```python
from build123d import *

# Parameters (mm, degrees)
F1_DEPTH = 1.5
F2_R     = 6
F3_R     = 20


with BuildPart() as f1:
    # F0 (on Top) → F1 (new body)
    with BuildSketch(Plane.XY):
        Polygon((16.235917, 84.775943), (-13.764083, 84.775943), (-13.764083, 61.775943), (-7.764083, 24.775943), (-7.764083, 9.775943), (-13.764083, -27.224057), (-13.764083, -50.224057), (16.235917, -50.224057), (16.235917, -27.224057), (10.235917, 9.775943), (10.235917, 24.775943), (16.235917, 61.775943), align=None)
        with BuildLine():
            ThreePointArc((-4.764083, -43.224057), (-4.471189, -42.51695), (-3.764083, -42.224057))
            Line((-3.764083, -42.224057), (6.235917, -42.224057))
            ThreePointArc((6.235917, -42.224057), (6.943024, -42.51695), (7.235917, -43.224057))
            ThreePointArc((7.235917, -43.224057), (6.943024, -43.931164), (6.235917, -44.224057))
            Line((6.235917, -44.224057), (-3.764083, -44.224057))
            ThreePointArc((-3.764083, -44.224057), (-4.471189, -43.931164), (-4.764083, -43.224057))
        make_face(mode=Mode.SUBTRACT)
        with BuildLine():
            Line((6.735917, 28.275943), (-3.764083, 28.275943))
            ThreePointArc((-3.764083, 28.275943), (-4.471189, 27.98305), (-4.764083, 27.275943))
            Line((-4.764083, 27.275943), (-4.764083, 19.275943))
            ThreePointArc((-4.764083, 19.275943), (-4.471189, 18.568836), (-3.764083, 18.275943))
            Line((-3.764083, 18.275943), (6.735917, 18.275943))
            ThreePointArc((6.735917, 18.275943), (7.089471, 18.129496), (7.235917, 17.775943))
            Line((7.235917, 17.775943), (7.235917, 17.275943))
            Line((7.235917, 17.275943), (7.235917, 16.775943))
            ThreePointArc((7.235917, 16.775943), (7.089471, 16.42239), (6.735917, 16.275943))
            Line((6.735917, 16.275943), (-3.764083, 16.275943))
            ThreePointArc((-3.764083, 16.275943), (-4.471189, 15.98305), (-4.764083, 15.275943))
            Line((-4.764083, 15.275943), (-4.764083, 7.275943))
            ThreePointArc((-4.764083, 7.275943), (-4.471189, 6.568836), (-3.764083, 6.275943))
            Line((-3.764083, 6.275943), (6.735917, 6.275943))
            ThreePointArc((6.735917, 6.275943), (7.089471, 6.129496), (7.235917, 5.775943))
            ThreePointArc((7.235917, 5.775943), (7.089471, 5.42239), (6.735917, 5.275943))
            Line((6.735917, 5.275943), (-4.764083, 5.275943))
            ThreePointArc((-4.764083, 5.275943), (-5.471189, 5.568836), (-5.764083, 6.275943))
            Line((-5.764083, 6.275943), (-5.764083, 16.775943))
            Line((-5.764083, 16.775943), (-5.764083, 17.775943))
            Line((-5.764083, 17.775943), (-5.764083, 28.275943))
            ThreePointArc((-5.764083, 28.275943), (-5.471189, 28.98305), (-4.764083, 29.275943))
            Line((-4.764083, 29.275943), (6.735917, 29.275943))
            ThreePointArc((6.735917, 29.275943), (7.089471, 29.129496), (7.235917, 28.775943))
            ThreePointArc((7.235917, 28.775943), (7.089471, 28.42239), (6.735917, 28.275943))
        make_face(mode=Mode.SUBTRACT)
        with BuildLine():
            Line((6.235917, 76.775943), (-3.764083, 76.775943))
            ThreePointArc((-3.764083, 76.775943), (-4.471189, 77.068836), (-4.764083, 77.775943))
            ThreePointArc((-4.764083, 77.775943), (-4.471189, 78.48305), (-3.764083, 78.775943))
            Line((-3.764083, 78.775943), (6.235917, 78.775943))
            ThreePointArc((6.235917, 78.775943), (6.943024, 78.48305), (7.235917, 77.775943))
            ThreePointArc((7.235917, 77.775943), (6.943024, 77.068836), (6.235917, 76.775943))
        make_face(mode=Mode.SUBTRACT)
    extrude(amount=F1_DEPTH)

    # F2
    f2_edges = [f1.edges().sort_by_distance(p)[0] for p in [
        (16.235917, 84.775943, 0.75),
        (-13.764083, 84.775943, 0.75),
        (-13.764083, -50.224057, 0.75),
        (16.235917, -50.224057, 0.75),
    ]]
    fillet(f2_edges, radius=F2_R)

    # F3
    f3_edges = [f1.edges().sort_by_distance(p)[0] for p in [
        (16.235917, 61.775943, 0.75),
        (-13.764083, 61.775943, 0.75),
        (16.235917, -27.224057, 0.75),
        (-13.764083, -27.224057, 0.75),
        (-7.764083, 9.775943, 0.75),
        (10.235917, 9.775943, 0.75),
        (10.235917, 24.775943, 0.75),
        (-7.764083, 24.775943, 0.75),
    ]]
    fillet(f3_edges, radius=F3_R)


solid = f1.part
```
Work out the finished part from the listing and answer in its coordinate system (mm). A direction names the side the tool comes from. Coordinates: 2 decimals unless noted, no trailing zeros. Loops run counter-clockwise (first coordinate to the right, second up) from the corner with the lowest first, then second, coordinate; pieces in that order, holes last. Notation, with made-up numbers: M -36.5,77.25 L -29.5,77.25 A9 ccw -29.5,90.25 Z; hole C -32.75,-3.75 d5. An arc over 180 degrees is marked long. Use CSV: the item, a comma, the result in double quotes. Start each with the question number.
(1) Find section D-D, the plane y = 51. Give the vertices of the cut face in (x, z), then the cut area to 3 significant figures.
(2) Find section A-A, the plane x = 0. Give the vertices of the cut face in (y, z).
(3) Find section C-C, the plane z = 0.25. State how many separate pieces and enclosed holes the cut face has, then the cut area to 3 significant figures.
(4) For a pull along Y with two mould halves and no side action, classify faces 1 (the face through (14.525, -48.42, 0.76)), 2 (the face through (-10.726, -8.487, 0.74)), 3 (the face through (14.432, 83.065, 0.76)) as +Y half, -Y half, draft (parallel to the pull), parting line (faces both ways), or undercut.
(5) Consider line 1 (Y direction, x = 3, z = 0.8); line 2 (X direction, y = -43, z = 1.4); line 3 (Y direction, x = -5, z = 1.3). Determine where each line is inside the solid, lowest interval first.
(6) Given pin 1 Ø0.8 at (y, z) = (21, 0.5) entering from +X; pin 2 Ø0.8 at (y, z) = (22.5, 0.5) entering from -X, each flat-ended and moving along its own axis, determine where each tip first touches the part or whether it passes through.
(7) For faces 4 (the face through (8, 18, 1.5)), 5 (the face through (13.198, 43.039, 0.74)), 6 (the face through (-10.8, 43.5, 0.7)), determine the directions among +Z, -Z, +X, -X, +Y, -Y from which every point of the face is accessible in a straight line to the end or side of a thin tool.
(8) Find section B-B, the plane x = 12.5. Give the vertices of the cut face in (y, z), then the cut area to 3 significant figures.
Recorded:
1,outline,"M -12.02,0 L 14.49,0 L 14.49,1.5 L -12.02,1.5 Z"
1,area,"39.8 mm^2"
2,outline,"M -50.22,0 L -44.22,0 L -44.22,1.5 L -50.22,1.5 Z; M -42.22,0 L 5.28,0 L 5.28,1.5 L -42.22,1.5 Z; M 6.28,0 L 16.28,0 L 16.28,1.5 L 6.28,1.5 Z; M 18.28,0 L 28.28,0 L 28.28,1.5 L 18.28,1.5 Z; M 29.28,0 L 76.78,0 L 76.78,1.5 L 29.28,1.5 Z; M 78.78,0 L 84.78,0 L 84.78,1.5 L 78.78,1.5 Z"
3,separate pieces,"1"
3,enclosed holes,"3"
3,area,"3,280 mm^2"
4,face 1,"-Y half"
4,face 2,"undercut"
4,face 3,"+Y half"
5,line 1,"y = -50.22 to -44.22, -42.22 to 5.28, 6.28 to 16.28, 18.28 to 28.28, 29.28 to 76.78, 78.78 to 84.78"
5,line 2,"x = -13.76 to -4.74, 7.21 to 16.24"
5,line 3,"y = -50.22 to 5.3, 29.25 to 84.78"
6,pin 1,"stops at x = 10.24"
6,pin 2,"stops at x = -7.76"
7,face 4,"+Z, +X, -X, +Y, -Y"
7,face 5,"+Z, -Z, +X"
7,face 6,"+Z, -Z, -X"
8,outline,"M -49.78,0 L -4.19,0 L -4.19,1.5 L -49.78,1.5 Z; M 38.74,0 L 84.33,0 L 84.33,1.5 L 38.74,1.5 Z"
8,area,"137 mm^2"
